from build123d import *

# Parameters (mm, degrees)
BOSS_EXTRUDE1_DEPTH = 10
CUT_EXTRUDE1_DEPTH  = 2


with BuildPart() as part:
    # Sketch2 → Boss-Extrude1 (new body)
    with BuildSketch(Plane.XY):
        Polygon((50, 35), (-50, 35), (-50, 0), (-20, 0), (-20, 19), (20, 19), (20, 0), (50, 0), align=None)
    extrude(amount=BOSS_EXTRUDE1_DEPTH)

    # Sketch3 → Cut-Extrude1 (cut)
    # profile 1 of 2: a face of its own
    with BuildSketch(Plane.XY.offset(10)):
        Polygon((23.142767448, 27.42405293), (26.665033073, 27.42405293), (26.665033073, 8.37405293), (24.955417689, 8.37405293), (24.955417689, 25.470206776), (22.024648458, 25.470206776), align=None)
    # profile 2 of 2: a face of its own
    with BuildSketch(Plane.XY.offset(10)):
        with BuildLine():
            Line((37.899648458, 7.885591391), (36.533482593, 8.835801728))
            Line((36.533482593, 8.835801728), (41.8302374, 16.578680334))
            add(Edge.make_bspline(
                [(41.8302374, 16.578680334), (41.492286397, 16.537352375), (40.826842028, 16.455975319), (40.156624373, 16.44102567), (39.826781872, 16.433668314)],
                knots=[0, 0, 0, 0, 1.015715272, 2, 2, 2, 2], degree=3))
            add(Edge.make_bspline(
                [(39.826781872, 16.433668314), (39.626800154, 16.438790459), (39.234253531, 16.448844781), (38.657138394, 16.528538052), (38.102589842, 16.651275176), (37.572078062, 16.834420543), (37.063609043, 17.062031081), (36.578292803, 17.344281398), (36.116782656, 17.676329928), (35.684035182, 18.056420925), (35.290452718, 18.47376861), (34.939805911, 18.915487181), (34.648389179, 19.386707821), (34.406309478, 19.877818016), (34.222719438, 20.395876512), (34.089029055, 20.934988247), (34.00672024, 21.498931612), (33.99692802, 21.882789824), (33.99195615, 22.077688747)],
                knots=[0, 0, 0, 0, 1.060718605, 2.082097864, 3.085795603, 4.069760067, 5.054557537, 6.03741023, 7.043284206, 8.066802108, 9.088538119, 10.083643548, 11.053783639, 12.022749082, 12.983451788, 13.964007469, 14.966251758, 16, 16, 16, 16], degree=3))
            add(Edge.make_bspline(
                [(33.99195615, 22.077688747), (34.001396431, 22.344218128), (34.019925787, 22.867361236), (34.169052003, 23.631722179), (34.414308992, 24.354460366), (34.756274871, 25.033675564), (35.186993855, 25.659597274), (35.704656324, 26.223524132), (36.306113615, 26.717435408), (36.977664319, 27.142000458), (37.703485761, 27.483458086), (38.463682314, 27.735131993), (39.252429168, 27.883170892), (39.786741772, 27.902688222), (40.055748218, 27.912514468)],
                knots=[0, 0, 0, 0, 1.022988612, 2.007919123, 2.978103895, 3.94594894, 4.918897164, 5.887013414, 6.875921846, 7.89917871, 8.930658928, 9.948724884, 10.967259574, 12, 12, 12, 12], degree=3))
            add(Edge.make_bspline(
                [(40.055748218, 27.912514468), (40.319663759, 27.902553152), (40.841135992, 27.882870531), (41.607974728, 27.73872207), (42.342439406, 27.495771037), (43.040458548, 27.160030769), (43.686740206, 26.739184114), (44.267905692, 26.237709063), (44.770692555, 25.655293265), (45.19427682, 25.006023055), (45.534292325, 24.308428486), (45.779614323, 23.580261708), (45.930629872, 22.826759525), (45.949659881, 22.316249601), (45.959263843, 22.058608218)],
                knots=[0, 0, 0, 0, 1.026385292, 2.028040595, 3.023318987, 4.028184125, 5.03290303, 6.015178782, 7.004435299, 8.016004309, 9.023023918, 10.015172535, 10.998308025, 12, 12, 12, 12], degree=3))
            add(Edge.make_bspline(
                [(45.959263843, 22.058608218), (45.952849931, 21.858617143), (45.939840916, 21.452985271), (45.848747588, 20.836688691), (45.69406058, 20.208304142), (45.518519191, 19.676419457), (45.34907125, 19.237134894), (45.189589376, 18.890144152), (45.012630369, 18.524921562), (44.806243945, 18.145296765), (44.584380587, 17.746430396), (44.333686525, 17.332323043), (44.059880484, 16.902419009), (43.864864438, 16.612602716), (43.765003025, 16.464197161)],
                knots=[0, 0, 0, 0, 1.179839688, 2.393009684, 3.667231171, 4.993948276, 5.694988576, 6.444077775, 7.246288328, 8.089075292, 8.993003841, 9.939041771, 10.944649915, 12, 12, 12, 12], degree=3))
            Line((43.765003025, 16.464197161), (37.899648458, 7.885591391))
        make_face()
        with BuildLine():
            add(Edge.make_bspline(
                [(40.14351865, 18.387514468), (40.295015213, 18.391653129), (40.589927518, 18.399709693), (41.021966817, 18.44874571), (41.429768552, 18.535689834), (41.814422066, 18.660438552), (42.179784204, 18.81096985), (42.520051647, 19.00262366), (42.835509171, 19.231314202), (43.128269174, 19.488271573), (43.388241801, 19.773752606), (43.61979744, 20.072549715), (43.816614242, 20.385974521), (43.972080079, 20.717952134), (44.099903268, 21.060401512), (44.188175591, 21.418837359), (44.237076034, 21.791392226), (44.245412177, 22.044477779), (44.249648458, 22.173091391)],
                knots=[0, 0, 0, 0, 1.163407946, 2.26475976, 3.333800367, 4.359385343, 5.366239384, 6.363380779, 7.350133999, 8.353570782, 9.349036268, 10.310270964, 11.253520213, 12.184142, 13.120487599, 14.056272588, 15.012232024, 16, 16, 16, 16], degree=3))
            add(Edge.make_bspline(
                [(44.249648458, 22.173091391), (44.246003544, 22.301758712), (44.238820795, 22.55531345), (44.181195635, 22.928419891), (44.079821206, 23.285978925), (43.943801568, 23.629948065), (43.764621417, 23.957501232), (43.549609587, 24.27275082), (43.294162968, 24.573697973), (43.000234715, 24.853264798), (42.683272362, 25.110972649), (42.345485925, 25.338408291), (41.989659596, 25.52902366), (41.617964216, 25.686316625), (41.229625345, 25.809062718), (40.824872781, 25.897331517), (40.401661216, 25.946163495), (40.114380216, 25.95444695), (39.967977785, 25.958668314)],
                knots=[0, 0, 0, 0, 0.972161553, 1.915763587, 2.844109794, 3.775983486, 4.705125789, 5.659731448, 6.655561913, 7.682237399, 8.721216875, 9.739758359, 10.754845918, 11.767244016, 12.7857855, 13.828538656, 14.893392813, 16, 16, 16, 16], degree=3))
            add(Edge.make_bspline(
                [(39.967977785, 25.958668314), (39.822848607, 25.954440131), (39.538106356, 25.946144469), (39.118657146, 25.897424338), (38.716641361, 25.808469088), (38.329427685, 25.686373481), (37.957743349, 25.529011926), (37.601933802, 25.338398303), (37.264068354, 25.111025002), (36.947409888, 24.853062027), (36.652962627, 24.574999267), (36.401907962, 24.271432461), (36.186404063, 23.957665221), (36.007470119, 23.629904483), (35.87138499, 23.285990557), (35.770028095, 22.928416741), (35.712398224, 22.555314271), (35.705216121, 22.301758988), (35.701571535, 22.173091391)],
                knots=[0, 0, 0, 0, 1.099389452, 2.15699305, 3.192601482, 4.213358962, 5.227959689, 6.245255729, 7.266013209, 8.307253147, 9.336162325, 10.327954924, 11.284637477, 12.215801273, 13.149702402, 14.080068371, 15.025723358, 16, 16, 16, 16], degree=3))
            add(Edge.make_bspline(
                [(35.701571535, 22.173091391), (35.704869504, 22.044377624), (35.711373703, 21.790530517), (35.774117816, 21.41755115), (35.879046739, 21.060019694), (36.019577993, 20.714459731), (36.204643791, 20.384231475), (36.431740735, 20.070900548), (36.697926636, 19.770915026), (36.99964319, 19.488935773), (37.329851323, 19.230116075), (37.682530756, 19.004072138), (38.051610011, 18.813177834), (38.438388315, 18.660008301), (38.839999326, 18.536936247), (39.260052541, 18.44890595), (39.697158805, 18.400180041), (39.993304563, 18.391776831), (40.14351865, 18.387514468)],
                knots=[0, 0, 0, 0, 0.952633368, 1.87876736, 2.791047057, 3.707742249, 4.635551637, 5.587206343, 6.568248508, 7.601284464, 8.641511608, 9.671105535, 10.699146789, 11.713763218, 12.747829548, 13.806491675, 14.887386225, 16, 16, 16, 16], degree=3))
        make_face(mode=Mode.SUBTRACT)
    extrude(amount=-CUT_EXTRUDE1_DEPTH, mode=Mode.SUBTRACT)


solid = part.part
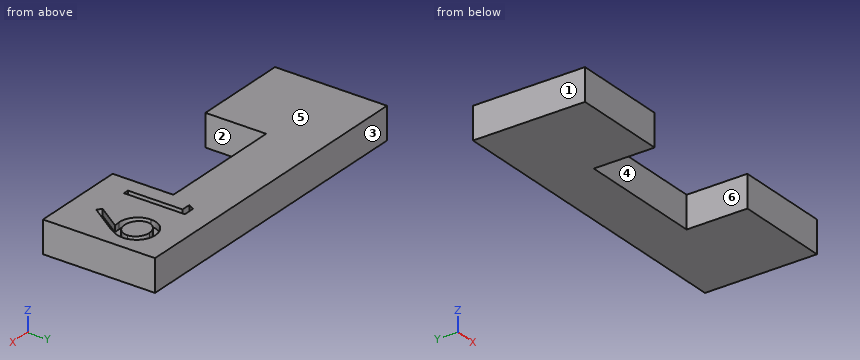
Here's how the part is built. I have some questions about the finished solid (model axes, mm). Face numbers are marked on the shaded views. A direction names the side the tool comes from. Coordinates: 2 decimals unless noted, no trailing zeros. Write each loop counter-clockwise with the first axis right and the second up, starting at its lowest first coordinate (ties: lowest second). Pieces come first, ordered by that corner, then holes. Notation, with made-up numbers: (-12.75, 74) - (-5.75, 74) arc R28 cw to (-5.75, 100) - close; hole circle Ø3 at (-4.75, 13). An arc over 180 degrees is marked (long way). Use one line per item in the form item = value.
1) Suppose I cut it at C-C, the plane x = 12. Write out the boundary of the cut face in (y, z).
Solved:
outline = (19, 0) - (35, 0) - (35, 10) - (19, 10) - close
2) Suppose I cut it at A-A, the plane y = 5. Write out the boundary of the cut face in (x, z), plus the area to 3 significant figures.
Solved:
outline = (-50, 0) - (-20, 0) - (-20, 10) - (-50, 10) - close; (20, 0) - (50, 0) - (50, 10) - (20, 10) - close
area = 600 mm2
3) Thinking about a two-plate mould opening in X: for the marked faces 1, 2, 3 and 4, which applies, released by +X, released by -X, zero draft, split by the parting line, or undercut?
Solved:
face_1 = released by -X
face_2 = undercut
face_3 = zero draft
face_4 = undercut
4) I need wall thicknesses on line 1 (X direction, y = 15.5, z = 3.5); line 2 (X direction, y = 20.5, z = 9.5); line 3 (Z direction, x = 38.5, y = 9.5). Which ranges of each line are inside material? Lowest first, please.
Solved:
line_1 = -50 to -20, 20 to 50
line_2 = -50 to 24.96, 26.67 to 34.2, 36.14 to 43.87, 45.76 to 50
line_3 = 0 to 8
5) On a 3-axis mill with a long thin cutter (end or side, diameter ignored), from which of +Z, -Z, +X, -X, +Y, -Y can I reach the whole of each face in a straight line? I mean the marked faces 5 and 6. Say none if no direction works.
Solved:
face_5 = +Z, +X, -X, +Y, -Y
face_6 = +Z, -Z, -Y
6) Suppose I cut it at D-D, the plane y = 11. Write out the boundary of the cut face in (x, z), plus the area to 3 significant figures.
Solved:
outline = (-50, 0) - (-20, 0) - (-20, 10) - (-50, 10) - close; (20, 0) - (50, 0) - (50, 10) - (40.03, 10) - (40.03, 8) - (38.01, 8) - (38.01, 10) - (26.67, 10) - (26.67, 8) - (24.96, 8) - (24.96, 10) - (20, 10) - close
area = 593 mm2
7) Suppose I cut it at B-B, the plane z = 4.75. Write out the boundary of the cut face in (x, y).
Solved:
outline = (-50, 0) - (-20, 0) - (-20, 19) - (20, 19) - (20, 0) - (50, 0) - (50, 35) - (-50, 35) - close
8) I'm going to push a flat-ended pin straight in: P1, Ø5, axis at x = -3, z = 6, coming from the -Y side. Where does the tip first touch, or does it pass through?
Solved:
P1 = 19
